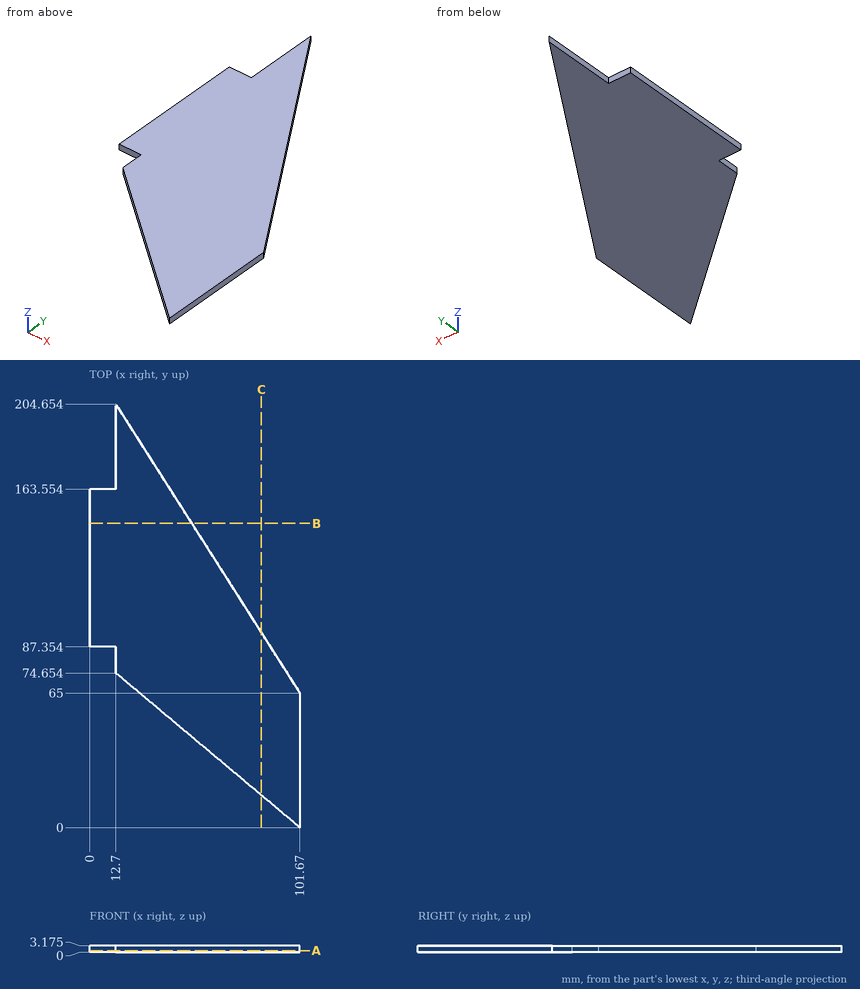
The figure shows three views and two pictorial views of one solid part (mm, origin at its lowest corner). Answer the questions. Give positions to 0.01 mm unless a question says otherwise; leave off trailing zeros. Order: outer loops, then holes, each group sorted by start corner. A loop starts at its lowest first (then second) coordinate and runs counter-clockwise, first axis right, second up. Notation, with made-up numbers: (67, -39) -> (82, -39) arc R32 cw to (82, -6) -> close; hole circle Ø5 at (-23, 1.5). An arc over 180 degrees is marked (long way). Answer as CSV lines item,"result". Start each with the question number.
(1) Each of these flat-tipped pins is pushed along its axis until it touches: pin 1 Ø1 at (x, z) = (8, 2.5) entering from -Y; pin 2 Ø1.6 at (x, z) = (4, 2) entering from +Y; pin 3 Ø1.6 at (y, z) = (83.5, 2) entering from -X. Where does it stop, or does it pass through?
(2) Section B-B, the plane y = 147 is taken. Write down the section's boundary in (x, z) (1 decimal).
(3) Section A-A, the plane z = 0.7 is taken. Write down the section's boundary in (x, y) (1 decimal).
(4) Consider line 1 along Y through (x, z) = (9, 2) (1 decimal); line 2 along Y through (x, z) = (53, 2.3) (1 decimal); line 3 along X through (y, z) = (84, 2.8) (1 decimal). Determine where each line is inside the solid, lowest interval first.
(5) Section C-C, the plane x = 83 is taken. Write down the section's boundary in (y, z) (1 decimal), plus the area to 3 significant figures.
Entries:
1,pin 1,"y = 87.35"
1,pin 2,"y = 163.55"
1,pin 3,"x = 12.7"
2,outline,"(0, 0) -> (49.4, 0) -> (49.4, 3.2) -> (0, 3.2) -> close"
3,outline,"(0, 87.4) -> (12.7, 87.4) -> (12.7, 74.7) -> (101.7, 0) -> (101.7, 65) -> (12.7, 204.7) -> (12.7, 163.6) -> (0, 163.6) -> close"
4,line 1,"87.4 to 163.6"
4,line 2,"40.8 to 141.4"
4,line 3,"12.7 to 89.6"
5,outline,"(15.7, 0) -> (94.3, 0) -> (94.3, 3.2) -> (15.7, 3.2) -> close"
5,area,"250 mm²"
